from build123d import *

# Parameters (mm, degrees)
BOSS_EXTRUDE1_DEPTH = 2
SKETCH3_R           = 1.325
CUT_EXTRUDE2_DEPTH  = 3
SKETCH6_R           = 2.5
BOSS_EXTRUDE2_DEPTH = 2
SKETCH7_R           = 1.325
CUT_EXTRUDE3_DEPTH  = 132.863565855


with BuildPart() as part:
    # Sketch1 → Boss-Extrude1 (new body)
    with BuildSketch(Plane(origin=(0, 0, 0), x_dir=(1, 0, 0), z_dir=(0, 1, 0))):
        with BuildLine():
            Line((-110, 20), (90, 20))
            ThreePointArc((90, 20), (70, 0), (90, -20))
            Line((90, -20), (-110, -20))
            ThreePointArc((-110, -20), (-130, 0), (-110, 20))
        make_face()
    extrude(amount=BOSS_EXTRUDE1_DEPTH)

    # Sketch3 → Cut-Extrude2 (cut)
    with BuildSketch(Plane(origin=(0, 2, 0), x_dir=(1, 0, 0), z_dir=(0, 1, 0))):
        with Locations(Location((69.75, -16.85, 0), (0, 0, 270))):
            Circle(SKETCH3_R)
        with Locations(Location((69.75, 16.85, 0), (0, 0, 270))):
            Circle(SKETCH3_R)
        with Locations(Location((-30.25, -16.85, 0), (0, 0, 270))):
            Circle(SKETCH3_R)
        with Locations(Location((-30.25, 16.85, 0), (0, 0, 270))):
            Circle(SKETCH3_R)
    extrude(amount=-CUT_EXTRUDE2_DEPTH, mode=Mode.SUBTRACT)

    # Sketch6 → Boss-Extrude2 (add)
    with BuildSketch(Plane(origin=(0, 2, 0), x_dir=(1, 0, 0), z_dir=(0, 1, 0))):
        with Locations((-110.25, -19.5)):
            Circle(SKETCH6_R)
        with Locations((-110.25, 19.5)):
            Circle(SKETCH6_R)
    extrude(amount=-BOSS_EXTRUDE2_DEPTH)

    # Sketch7 → Cut-Extrude3 (cut, through all)
    with BuildSketch(Plane(origin=(0, 2, 0), x_dir=(1, 0, 0), z_dir=(0, 1, 0))):
        with Locations(Location((-110.25, 19.5, 0), (0, 0, 270))):
            Circle(SKETCH7_R)
        with Locations(Location((-110.25, -19.5, 0), (0, 0, 270))):
            Circle(SKETCH7_R)
    extrude(amount=-CUT_EXTRUDE3_DEPTH, mode=Mode.SUBTRACT)


solid = part.part
Model file for the job. Use its own axes, mm. Give positions to 0.01 mm unless a question says otherwise; leave off trailing zeros. Loops run counter-clockwise (first coordinate to the right, second up) from the corner with the lowest first, then second, coordinate; pieces in that order, holes last. Notation, with made-up numbers: (-32, 56.25) - (9, 56.25) arc R23 cw to (9, 87.25) - close; hole circle Ø5 at (45.5, -31). An arc over 180 degrees is marked (long way). Use one line per item in the form item = value.
(1) Pull direction Z, two halves, no side cores. Call faces 1 (the face through (-18, 0, 0)), 2 (the face through (-130, 1, 0)), 3 (the face through (70, 1, 0)): pulls with the +Z half, pulls with the -Z half, needs draft (parallel to the pull), parting line crosses it, or undercut.
Determined:
face_1 = needs draft
face_2 = parting line crosses it
face_3 = undercut
(2) Cut at B-B (x = -54.5). Give the cut face in (y, z), then the cut area to 3 significant figures.
Determined:
outline = (0, -20) - (2, -20) - (2, 20) - (0, 20) - close
area = 80.0 mm^2
(3) Cut at A-A (y = 0.7). Give the cut face in (x, z) (3 decimals).
Determined:
outline = (-112.73, -19.813) arc R2.5 ccw to (-107.801, -20) - (90, -20) arc R20 cw to (90, 20) - (-107.801, 20) arc R2.5 ccw to (-112.73, 19.813) arc R20 ccw to start; hole circle Ø2.65 at (-110.25, -19.5); hole circle Ø2.65 at (-110.25, 19.5); hole circle Ø2.65 at (-30.25, -16.85); hole circle Ø2.65 at (-30.25, 16.85); hole circle Ø2.65 at (69.75, -16.85); hole circle Ø2.65 at (69.75, 16.85)
(4) Cut at C-C (z = 12.5). Give the cut face in (x, y), then the cut area to 3 significant figures.
Determined:
outline = (-125.61, 0) - (74.39, 0) - (74.39, 2) - (-125.61, 2) - close
area = 400 mm^2
(5) Drill centre lines: L1, parallel to Z at x = 69.75, y = 0.5 (3 decimals); L2, parallel to Z at x = -110.25, y = 1.1 (3 decimals); L3, parallel to X at y = 0.5, z = -16.85 (3 decimals). Where is each one in solid material? Low to high.
Determined:
L1 = -20 to -18.175, -15.525 to 15.525, 18.175 to 20
L2 = -22 to -20.825, -18.175 to 18.175, 20.825 to 22
L3 = -120.774 to -31.575, -28.925 to 68.425, 71.075 to 79.226
(6) Drop a flat-ended pin along its axis: P1, Ø1, axis at x = 20.5, y = 0.5, coming from the -Z side. Give the stop position or say it passes through.
Determined:
P1 = -20
